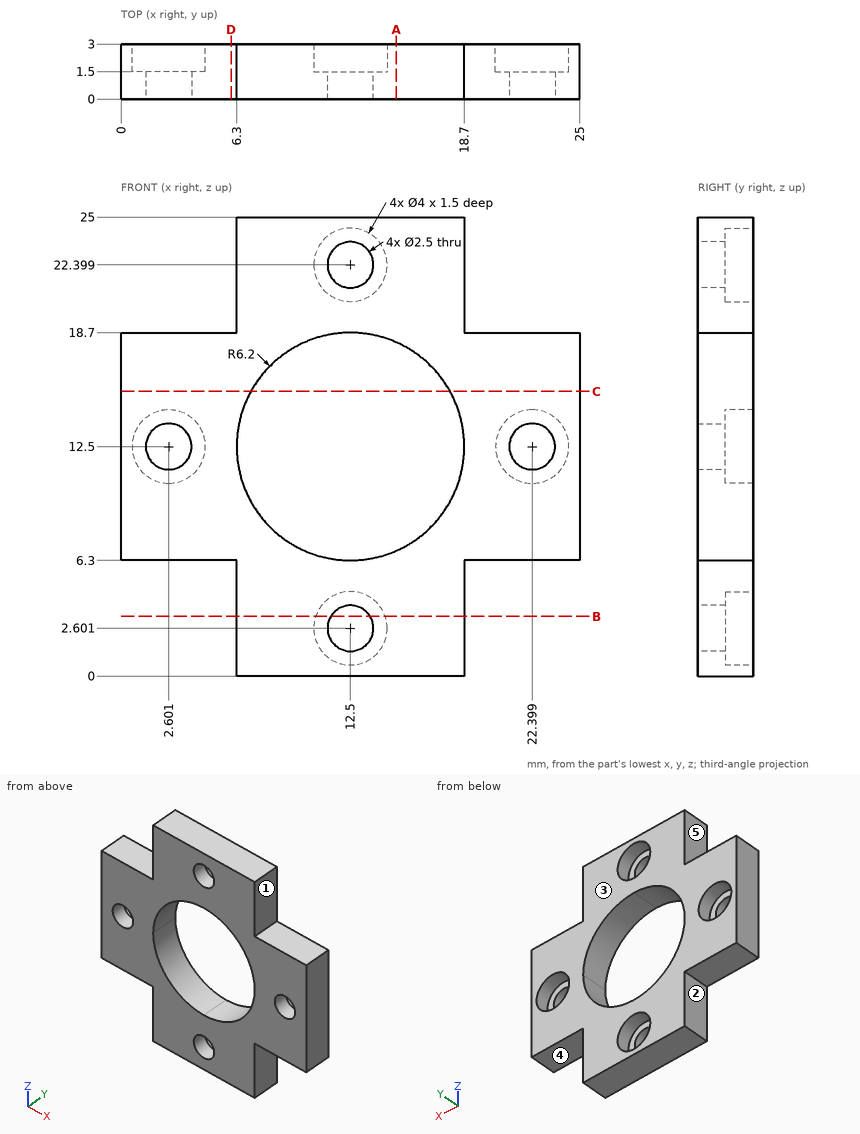
Geometry: see drawing. Coordinates: mm, zero at the bounding-box minimum. A direction names the side the tool comes from. Coordinates: 2 decimals unless noted, no trailing zeros. Write each loop counter-clockwise with the first axis right and the second up, starting at its lowest first coordinate (ties: lowest second). Pieces come first, ordered by that corner, then holes.
1) Section C-C on z = 15.5. Output: boundary loops of the cut face in (x, y) (1 decimal).
2) Material intervals for line 1 along X through (y, z) = (2.2, 12.5); line 2 along Z through (x, y) = (12, 0.35) (1 decimal), sorted ascending.
3) Section B-B on z = 3.25. Output: boundary loops of the cut face in (x, y).
4) Section D-D on x = 6. Output: boundary loops of the cut face in (y, z).
5) Section A-A on x = 15. Output: boundary loops of the cut face in (y, z).
6) Pin query (flat end, axial travel): pin 1 Ø0.9 at (x, y) = (3.5, 1.5) entering from -Z; pin 2 Ø1.5 at (y, z) = (1.5, 2.5) entering from -X; pin 3 Ø0.9 at (x, y) = (4, 2) entering from +Z. Return the tip coordinate at first contact, or that it passes through.
7) Set-up query: the marked faces 1, 2, 3, 4 and 5. Return all of +Z, -Z, +X, -X, +Y, -Y with unobstructed straight access to the full face (end or side cutting, diameter ignored); none if empty.
Check result:
1. outline: (0, 0) - (7.1, 0) - (7.1, 3) - (0, 3) - close; (17.9, 0) - (25, 0) - (25, 3) - (17.9, 3) - close
2. line 1: x = 0 to 0.6, 4.6 to 6.3, 18.7 to 20.4, 24.4 to 25
2. line 2: z = 0 to 1.5, 3.7 to 6.3, 18.7 to 21.3, 23.5 to 25
3. outline: (6.3, 0) - (11.43, 0) - (11.43, 1.5) - (10.61, 1.5) - (10.61, 3) - (6.3, 3) - close; (13.57, 0) - (18.7, 0) - (18.7, 3) - (14.39, 3) - (14.39, 1.5) - (13.57, 1.5) - close
4. outline: (0, 6.3) - (3, 6.3) - (3, 18.7) - (0, 18.7) - close
5. outline: (0, 0) - (3, 0) - (3, 6.83) - (0, 6.83) - close; (0, 18.17) - (3, 18.17) - (3, 25) - (0, 25) - close
6. pin 1: stops at z = 6.3
6. pin 2: stops at x = 6.3
6. pin 3: stops at z = 18.7
7. face 1: +Z, +X, +Y, -Y
7. face 2: -Z, -X, +Y, -Y
7. face 3: +Z, -Z, +X, -X, +Y
7. face 4: -Z, +X, +Y, -Y
7. face 5: +Z, -X, +Y, -Y
